Input: part model. Units: mm. Frame: model coordinates. A direction names the side the tool comes from. Coordinates: 2 decimals unless noted, no trailing zeros. Order: outer loops, then holes, each group sorted by start corner. A loop starts at its lowest first (then second) coordinate and runs counter-clockwise, first axis right, second up.
Autodesk Fusion 360 part; units mm, degrees
sketch "Sketch1" plane through (0, 0, 0) normal (0, 1, 0) x (1, 0, 0)
  circle A0 centre (0, 0) radius 28.5
  line L0 (-9, 27.0416) -> (9, 27.0416)
  line L1 (-27.3663, -7.9584) -> (-39.2742, -7.9584)
  line L2 (-49.2742, 2.0416) -> (-49.2742, 27.0416)
  line L3 (-49.2742, 27.0416) -> (-9, 27.0416)
  line L4 (-41.2742, 27.0416) -> (-34.2742, 27.0416)
  line L5 (-34.2742, 27.0416) -> (-34.2742, 2.0416)
  line L6 (-34.2742, 2.0416) -> (-41.2742, 2.0416)
  line L7 (-41.2742, 2.0416) -> (-41.2742, 27.0416)
  line L8 (-41.2742, 2.0416) -> (-49.2742, 2.0416)
  line L9 (-49.2742, 2.0416) -> (-34.2742, 2.0416)
  line L10 (-28.4268, 2.0416) -> (-34.2742, 2.0416)
  line L11 (-44.2742, 11.0416) -> (-31.2742, 11.0416)
  line L12 (-31.2742, 11.0416) -> (-31.2742, 18.0416)
  line L13 (-31.2742, 18.0416) -> (-44.2742, 18.0416)
  line L14 (-44.2742, 18.0416) -> (-44.2742, 11.0416)
  line L15 (-37.7742, 18.0416) -> (-37.7742, 27.0416)
  line L16 (-44.2742, 14.5416) -> (-41.2742, 14.5416)
  line L17 (-44.2742, 11.0416) -> (-49.2742, 11.0416)
  line L18 (-31.2742, 11.0416) -> (-26.2742, 11.0416)
  arc A1 (-49.2742, 2.0416) -> (-39.2742, -7.9584) centre (-39.2742, 2.0416) ccw
  line L19 (0, 27.0416) -> (0, 0)
  line L20 (27.3663, -7.9584) -> (39.2742, -7.9584)
  arc A2 (39.2742, -7.9584) -> (49.2742, 2.0416) centre (39.2742, 2.0416) ccw
  line L21 (49.2742, 2.0416) -> (49.2742, 27.0416)
  line L22 (49.2742, 27.0416) -> (9, 27.0416)
  line L23 (31.2742, 18.0416) -> (44.2742, 18.0416)
  line L24 (31.2742, 11.0416) -> (31.2742, 18.0416)
  line L25 (44.2742, 11.0416) -> (31.2742, 11.0416)
  line L26 (44.2742, 18.0416) -> (44.2742, 11.0416)
  line L27 (41.2742, 2.0416) -> (41.2742, 27.0416)
  line L28 (34.2742, 27.0416) -> (34.2742, 2.0416)
  line L29 (34.2742, 2.0416) -> (41.2742, 2.0416)
  circle A3 centre (0, 0) radius 1
  circle A4 centre (0, 0) radius 7.5
  line L30 (0, 0) -> (-7.5, 0)
  line L31 (-7.5, 0) -> (-7.5, 27.0416)
  line L32 (0, 0) -> (7.5, 0)
  line L33 (7.5, 0) -> (7.5, 27.0416)
  line L34 (-2, 27.0416) -> (2, 27.0416)
  line L35 (2, 27.0416) -> (2, 12.0416)
  line L36 (2, 12.0416) -> (-2, 12.0416)
  line L37 (-2, 12.0416) -> (-2, 27.0416)
  line L38 (-3.5, 18.0416) -> (3.5, 18.0416)
  line L39 (3.5, 18.0416) -> (3.5, 21.0416)
  line L40 (3.5, 21.0416) -> (-3.5, 21.0416)
  line L41 (-3.5, 21.0416) -> (-3.5, 18.0416)
  line L42 (-2, 19.5416) -> (-3.5, 19.5416)
  line L43 (-7.5, 27.0416) -> (-4.5, 27.0416)
  line L44 (-4.5, 27.0416) -> (-4.5, 32.0416)
  line L45 (-4.5, 32.0416) -> (-7.5, 32.0416)
  line L46 (-7.5, 32.0416) -> (-7.5, 27.0416)
  line L47 (7.5, 27.0416) -> (4.5, 27.0416)
  line L48 (4.5, 27.0416) -> (4.5, 32.0416)
  line L49 (4.5, 32.0416) -> (7.5, 32.0416)
  line L50 (7.5, 32.0416) -> (7.5, 27.0416)
  point P0 (0, 21.0416)
  point P1 (0, 27.0416)
  dimension "d1" = 57
  dimension "d2" = 18
  dimension "d3" = 25
  dimension "d4" = 90
  dimension "d5" = 10
  dimension "d8" = 7
  dimension "d9" = 7
  dimension "d10" = 13
  dimension "d11" = 90
  dimension "d12" = 90
  dimension "d13" = 5
  dimension "d14" = 5
  dimension "d15" = 10
  dimension "d18" = 2
  dimension "d19" = 15
  dimension "d20" = 4
  dimension "d21" = 15
  dimension "d22" = 3
  dimension "d23" = 7
  dimension "d24" = 90
  dimension "d25" = 5
  dimension "d26" = 5
  dimension "d27" = 3
  dimension "d28" = 3
extrude "Extrude1" add sketch "Sketch1" along normal blind 100 contours A0 L0 L47 L48 L50 | A0 L48 L49 L50 | L0 L19 A4 L33 L35 L36 L38 L39 L40 L47 | L19 A3 A4 L32 | A3 A4 L30 L32 | A0 L0 L43 L44 L46 | A0 L44 L45 L46 | L0 L19 A4 L31 L36 L37 L38 L40 L41 L43 | L19 A3 A4 L30
sketch "Sketch2" plane through (7.5, 0, 0) normal (1, 0, 0) x (0, 1, 0)
  line L0 (0, 0) -> (0, -32.0416)
  line L1 (0, -32.0416) -> (100, -32.0416)
  line L2 (100, -32.0416) -> (100, 0)
  line L3 (100, 0) -> (0, 0)
  line L4 (5, 16.673) -> (106.6592, 16.673)
  line L5 (106.6592, 16.673) -> (106.6592, -53.0106)
  line L6 (106.6592, -53.0106) -> (5, -53.0106)
  line L7 (5, -53.0106) -> (5, 16.673)
  dimension "d29" = 5
extrude "Extrude2" cut sketch "Sketch2" against normal blind 100 contours L1 L2 L3 L4 L5 L6 L7 | L1 L2 L3 L7
extrude "Extrude3" add 1 faces at (-3.3745, 0, -4.2745) along direction (0, -1, 0) blind 1
Item 1: Cut plane B-B on y = 2.85. Return loops of the section in (x, z), then the cut area to 3 significant figures.
Response values:
outline: (-7.5, -32.04) - (-4.5, -32.04) - (-4.5, -27.04) - (-2, -27.04) - (-2, -21.04) - (-3.5, -21.04) - (-3.5, -18.04) - (-2, -18.04) - (-2, -12.04) - (2, -12.04) - (2, -18.04) - (3.5, -18.04) - (3.5, -21.04) - (2, -21.04) - (2, -27.04) - (4.5, -27.04) - (4.5, -32.04) - (7.5, -32.04) - (7.5, 0) arc R7.5 ccw to (-7.5, 0) - close; hole circle Ø2 at (0, 0)
area: 452 mm2
Item 2: Access query for faces 5 (the face through (0, 2, -12.042)), 6 (the face through (3, 2, -21.042)), 7 (the face through (6, 2, -32.042)). Directions: +Z, -Z, +X, -X, +Y, -Y. A direction counts if a zero-diameter tool reaches every point of the face in a straight line with its end or side. Return the directions, or none.
Response values:
face 5: -Z, +Y, -Y
face 6: +Y, -Y
face 7: -Z, +X, -X, +Y, -Y
Item 3: Cut plane A-A on x = 0. Return loops of the section in (y, z), then the cut area to 3 significant figures.
Response values:
outline: (-1, -12.04) - (5, -12.04) - (5, -1) - (-1, -1) - close; (-1, 1) - (5, 1) - (5, 7.5) - (-1, 7.5) - close
area: 105 mm2
Item 4: Draft query along Z for faces 1 (the face through (-3.5, 2, -20)), 2 (the face through (0, -1, -8)), 3 (the face through (3.5, 2, -20)), 4 (the face through (-3, 2, -27.042)). Return one class per face: pulls with the +Z half, pulls with the -Z half, needs draft (parallel to the pull), parting line crosses it, or undercut.
Response values:
face 1: undercut
face 2: needs draft
face 3: undercut
face 4: pulls with the -Z half
Item 5: Pin query (flat end, axial travel): pin 1 Ø0.8 at (x, y) = (-3, 3) entering from +Z; pin 2 Ø2.5 at (x, z) = (0, 0) entering from -Y; pin 3 Ø0.8 at (x, y) = (-2.5, 1) entering from -Z; pin 4 Ø1.6 at (x, y) = (3, 1.5) entering from +Z. Return the tip coordinate at first contact, or that it passes through.
Response values:
pin 1: stops at z = 7.03
pin 2: stops at y = -1
pin 3: stops at z = -27.04
pin 4: stops at z = 7.17
Item 6: Ray query, probe 1 along X at (y, z) = (3.95, -15); probe 2 along Z at (x, y) = (0, 1.55); probe 3 along X at (y, z) = (1.9, 0). Return the intervals inside material, ascending.
Response values:
probe 1: x = -7.5 to -2, 2 to 7.5
probe 2: z = -12.04 to -1, 1 to 7.5
probe 3: x = -7.5 to -1, 1 to 7.5
Item 7: Cut plane C-C on z = 1.5. Return loops of the section in (x, y), then the cut area to 3 significant figures.
Response values:
outline: (-7.35, -1) - (7.35, -1) - (7.35, 5) - (-7.35, 5) - close
area: 88.2 mm2
